Part print with two shaded views. Sizes in mm from the minimum x, y, z corner. Round coordinates to 2 decimals unless told otherwise and drop trailing zeros. Loops run counter-clockwise (first coordinate to the right, second up) from the corner with the lowest first, then second, coordinate; pieces in that order, holes last. Notation, with made-up numbers: (58, -35.5) - (75, -35.5) arc R31 ccw to (75, -7.5) - close; hole circle Ø7 at (76, 17.25). An arc over 180 degrees is marked (long way). One line per question, with ' | ' between items.
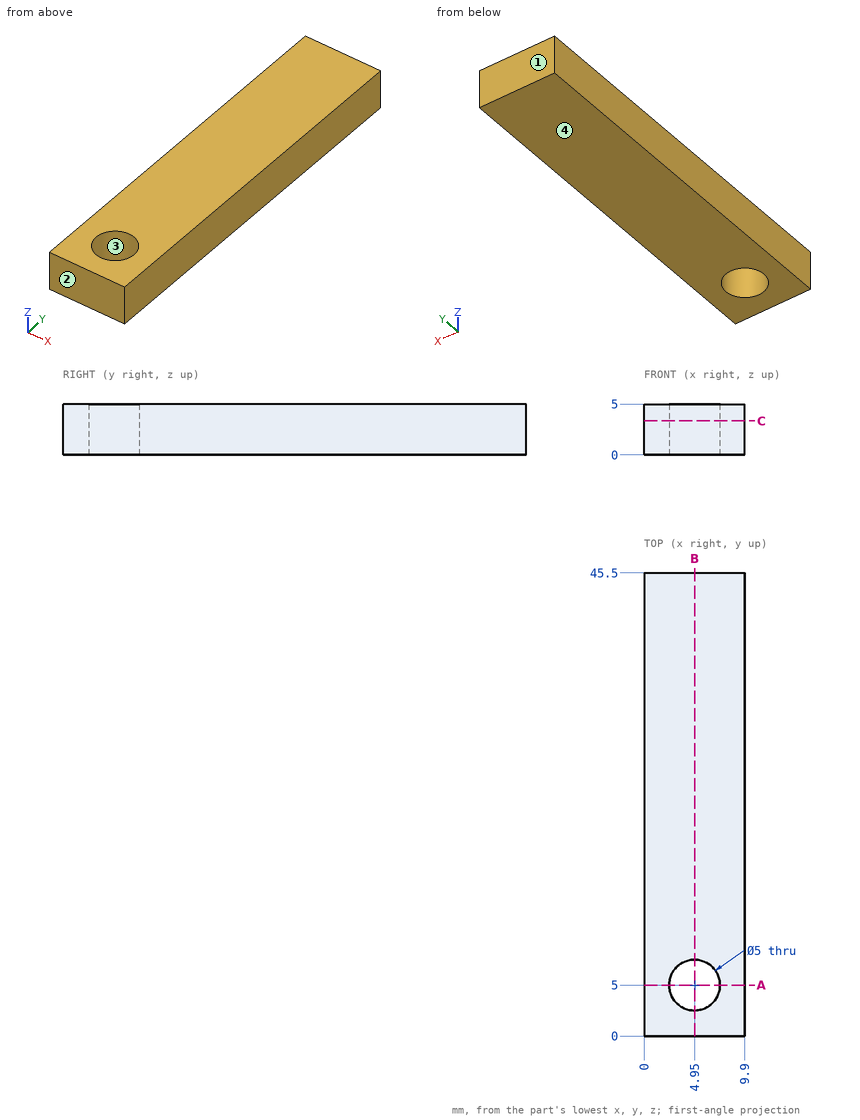
(1) Probe L1, parallel to X at y = 5, z = 1.2; L2, parallel to Y at x = 4.95, z = 3.65; L3, parallel to Y at x = 3.75, z = 0.65. List the from-to ranges inside material, lowest first.
Results found:
L1: x = 0 to 2.45, 7.45 to 9.9 | L2: y = 0 to 2.5, 7.5 to 45.5 | L3: y = 0 to 2.81, 7.19 to 45.5
(2) Two-plate mould, pull along Y, no slides. Class the marked faces 1, 2, 3 and 4: released by +Y, released by -Y, zero draft, split by the parting line, or undercut.
Results found:
face 1: released by +Y | face 2: released by -Y | face 3: undercut | face 4: zero draft
(3) Cut at B-B, the plane x = 4.95. Write the cut outline in (y, z).
Results found:
outline: (0, 0) - (2.5, 0) - (2.5, 5) - (0, 5) - close; (7.5, 0) - (45.5, 0) - (45.5, 5) - (7.5, 5) - close
(4) Cut at C-C, the plane z = 3.35. Write the cut outline in (x, y), then the cut area to 3 significant figures.
Results found:
outline: (0, 0) - (9.9, 0) - (9.9, 45.5) - (0, 45.5) - close; hole circle Ø5 at (4.95, 5) | area: 431 mm²
(5) Cut at A-A, the plane y = 5. Write the cut outline in (x, z).
Results found:
outline: (0, 0) - (2.45, 0) - (2.45, 5) - (0, 5) - close; (7.45, 0) - (9.9, 0) - (9.9, 5) - (7.45, 5) - close
